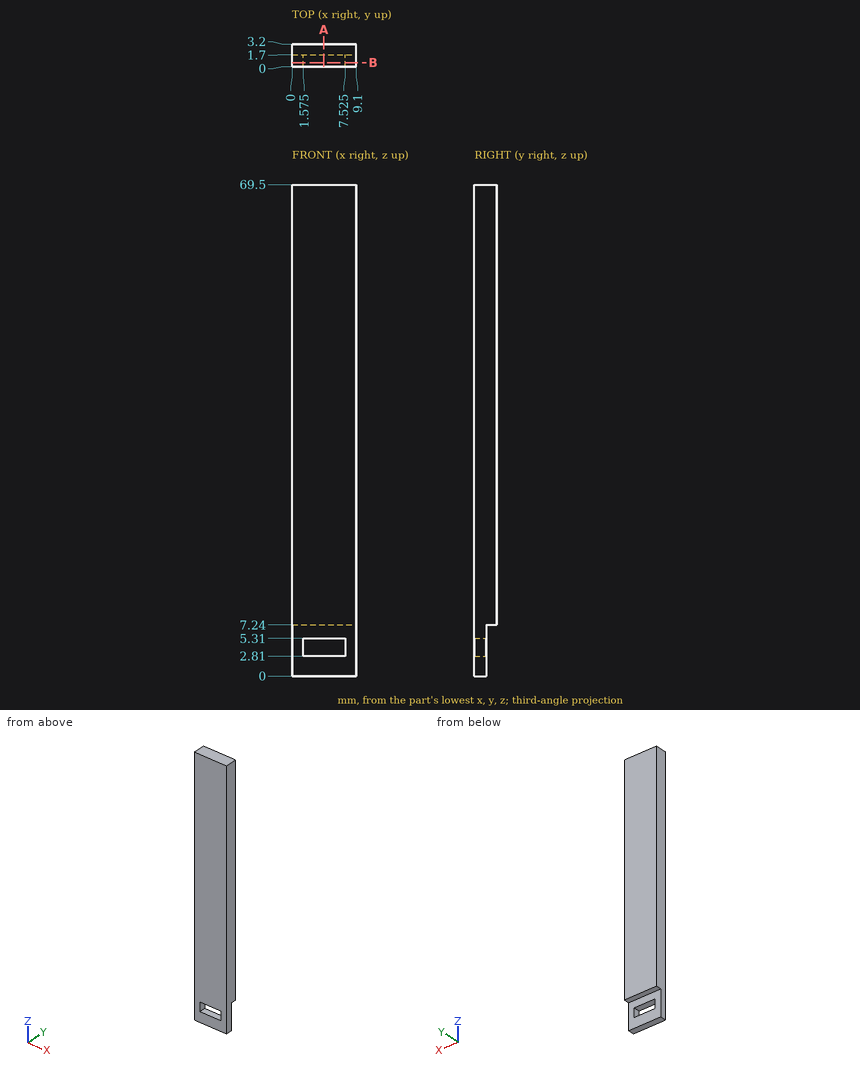
Design review of the part shown in the three views and the two pictorial views. Dimensions are in mm from the part's minimum x, y and z. Round coordinates to 2 decimals unless told otherwise and drop trailing zeros. Order: outer loops, then holes, each group sorted by start corner. A loop starts at its lowest first (then second) coordinate and runs counter-clockwise, first axis right, second up.
Item 1: To check wall thickness, follow probe 1 along Z at (x, y) = (5, 1.2); probe 2 along Y at (x, z) = (1.5, 6); probe 3 along Z at (x, y) = (4, 2.9). State the ranges of each line that lie inside material, in increasing order.
Working result:
probe 1: z = 0 to 2.81, 5.31 to 69.5
probe 2: y = 0 to 1.7
probe 3: z = 7.24 to 69.5
Item 2: Add section A-A, the plane x = 4.5. State the section outline as (y, z) points, and give its area (3 significant figures).
Working result:
outline: (0, 0) - (1.7, 0) - (1.7, 2.81) - (0, 2.81) - close; (0, 5.31) - (1.7, 5.31) - (1.7, 7.24) - (3.2, 7.24) - (3.2, 69.5) - (0, 69.5) - close
area: 207 mm2
Item 3: Add section B-B, the plane y = 0.55. State the section outline as (x, z) points (3 decimals).
Working result:
outline: (0, 0) - (9.1, 0) - (9.1, 69.5) - (0, 69.5) - close; hole (1.575, 2.81) - (7.525, 2.81) - (7.525, 5.31) - (1.575, 5.31) - close
